```python
from build123d import *

# Parameters (mm, degrees)
EXTRUDE_1_DEPTH              = 14
SKETCH_2_R                   = 38
EXTRUDE_2_DEPTH              = 6
SKETCH_3_R                   = 31
EXTRUDE_3_DEPTH              = 28
SKETCH_4_R                   = 20
CUT_EXTRUDE_4_DEPTH          = 88.8179936
SKETCH_5_R                   = 2.5
CUT_EXTRUDE_5_DEPTH          = 79.689262292
HOLE_WIZARD_M8_1_D           = 9
HOLE_WIZARD_M8_1_CBORE_D     = 15
HOLE_WIZARD_M8_1_CBORE_DEPTH = 8
FILLET_1_R                   = 14


with BuildPart() as part:
    # 草圖1 → 伸長1 (new body)
    with BuildSketch(Plane(origin=(0, 0, 0), x_dir=(0, 0, -1), z_dir=(1, 0, 0))):
        with BuildLine():
            ThreePointArc((41.00892786, 41.00892786), (0, 52), (-41.00892786, 41.00892786))
            ThreePointArc((-41.00892786, 41.00892786), (-52, 0), (-41.00892786, -41.00892786))
            ThreePointArc((-41.00892786, -41.00892786), (0, -52), (41.00892786, -41.00892786))
            ThreePointArc((41.00892786, -41.00892786), (52, 0), (41.00892786, 41.00892786))
        make_face()
    extrude(amount=EXTRUDE_1_DEPTH)

    # 草圖2 → 伸長2 (add)
    with BuildSketch(Plane(origin=(14, 0, 0), x_dir=(0, 0, -1), z_dir=(1, 0, 0))):
        Circle(SKETCH_2_R)
    extrude(amount=EXTRUDE_2_DEPTH)

    # 草圖3 → 伸長3 (add)
    with BuildSketch(Plane.ZY):
        with Locations(Location((0, 0, 0), (0, 0, 180))):
            Circle(SKETCH_3_R)
    extrude(amount=EXTRUDE_3_DEPTH)

    # 草圖4 → 伸長4 (cut, through all)
    with BuildSketch(Plane(origin=(20, 0, 0), x_dir=(0, 0, -1), z_dir=(1, 0, 0))):
        Circle(SKETCH_4_R)
    extrude(amount=-CUT_EXTRUDE_4_DEPTH, mode=Mode.SUBTRACT)

    # 草圖5 → 伸長5 (cut, through all)
    with BuildSketch(Plane(origin=(0, 0, 0), x_dir=(1, 0, 0), z_dir=(0, 1, 0))):
        with Locations(Location((-18, 0, 0), (0, 0, 90))):
            Circle(SKETCH_5_R)
    extrude(amount=CUT_EXTRUDE_5_DEPTH, mode=Mode.SUBTRACT)

    # M8 六角承窩頭蓋螺釘的柱孔1 (through all)
    with Locations(Plane(origin=(20, 0, 0), x_dir=(0, 0, -1), z_dir=(1, 0, 0))):
        with Locations((29.69848481, 29.69848481), (29.69848481, -29.69848481), (-29.69848481, 29.69848481), (-29.69848481, -29.69848481)):
            CounterBoreHole(HOLE_WIZARD_M8_1_D / 2, HOLE_WIZARD_M8_1_CBORE_D / 2, HOLE_WIZARD_M8_1_CBORE_DEPTH)

    # 圓角1
    fillet_1_edges = [part.edges().sort_by_distance(p)[0] for p in [
        (7, 41.00892786, 41.00892786),
        (7, 41.00892786, -41.00892786),
        (7, -41.00892786, -41.00892786),
        (7, -41.00892786, 41.00892786),
    ]]
    fillet(fillet_1_edges, radius=FILLET_1_R)


solid = part.part
```
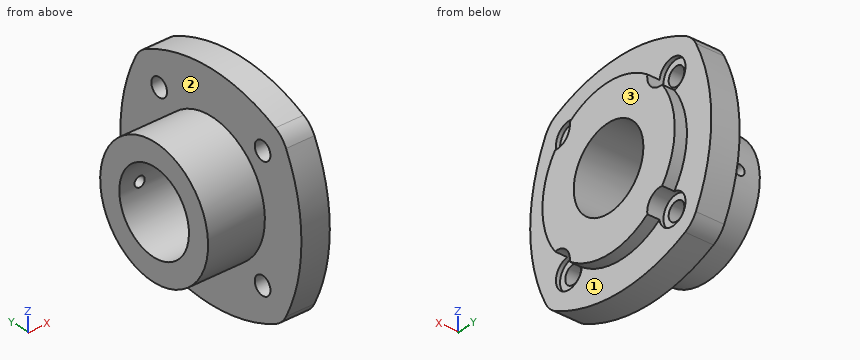
Could you check a few things on this model? Use its own coordinates, in mm. Face numbers are marked on the shaded views. A direction names the side the tool comes from. Give positions to 0.01 mm unless a question says otherwise; leave off trailing zeros. Loops run counter-clockwise (first coordinate to the right, second up) from the corner with the lowest first, then second, coordinate; pieces in that order, holes last. Notation, with made-up numbers: (50, -15.75) - (60, -15.75) arc R35 cw to (60, 16.25) - close; hole circle Ø2 at (-31.5, 80). An arc over 180 degrees is marked (long way). Answer in a Markdown table with one row per item. Add a question column.
Q1. Which directions (+Z, -Z, +X, -X, +Y, -Y) give clear straight access to the entire face, cutting with the end or side of a thin tool? Please do the marked faces 1, 2 and 3.
Q2. If we section it at A-A (y = 0): List the corners of the cut face in (x, z) for me.
Q3. Please list where these lines run through material, in increasing order: L1, parallel to Z at x = 7, y = -0.5; L2, parallel to Y at x = -3, z = 0; L3, parallel to X at y = 28, z = 0. Write a range as from..to.
Q4. If we section it at B-B (z = 0): List the corners of the cut face in (x, y) for me.
Q5. If we section it at C-C (y = -27.5): List the corners of the cut face in (x, z) for me, plus the area to 3 significant figures.
Q6. For pin 1 (12 mm diameter, centred on x = 1, y = 17, fed in from -Z); pin 2 (8 mm diameter, centred on x = -2.5, y = -39, fed in from -Z); pin 3 (11.5 mm diameter, centred on y = 29.7, z = 29.7, fed in from -X), each with a flat end and sliding along its axis, tell me the tip position at first contact or that it passes through.
Q7. If we section it at D-D (z = -17.5): List the corners of the cut face in (x, y) for me, plus the area to 3 significant figures.
The answers:
| question | item | result |
|---|---|---|
| 1 | face 1 | +X |
| 1 | face 2 | -X |
| 1 | face 3 | +Z, -Z, +X, +Y, -Y |
| 2 | outline | (-28, -31) - (0, -31) - (0, -52) - (14, -52) - (14, -38) - (20, -38) - (20, -20) - (-28, -20) - close; (-28, 20) - (20, 20) - (20, 38) - (14, 38) - (14, 52) - (0, 52) - (0, 31) - (-28, 31) - close |
| 3 | L1 | z = -52..-19.99, 19.99..52 |
| 3 | L2 | y = -31..-20, 20..31 |
| 3 | L3 | x = -28..-20.5, -15.5..20 |
| 4 | outline | (-28, -31) - (0, -31) - (0, -52) - (14, -52) - (14, -38) - (20, -38) - (20, -20) - (-28, -20) - close; (-28, 20) - (-20.5, 20) - (-20.5, 31) - (-28, 31) - close; (-15.5, 20) - (20, 20) - (20, 38) - (14, 38) - (14, 52) - (0, 52) - (0, 31) - (-15.5, 31) - close |
| 5 | outline | (-28, -14.31) - (0, -14.31) - (0, -25.77) - (12, -25.77) - (12, -22.53) - (20, -22.53) - (20, 22.53) - (12, 22.53) - (12, 25.77) - (0, 25.77) - (0, 14.31) - (-28, 14.31) - close; (0, -47.25) - (14, -47.25) - (14, -36.87) - (12, -36.87) - (12, -33.62) - (0, -33.62) - close; (0, 33.62) - (12, 33.62) - (12, 36.87) - (14, 36.87) - (14, 47.25) - (0, 47.25) - close |
| 5 | area | 2,150 mm^2 |
| 6 | pin 1 | stops at z = -51.26 |
| 6 | pin 2 | stops at z = -43.73 |
| 6 | pin 3 | stops at x = 0 |
| 7 | outline | (-28, -25.59) - (0, -25.59) - (0, -50.11) - (14, -50.11) - (14, -33.73) - (20, -33.73) - (20, -9.68) - (-28, -9.68) - close; (-28, 9.68) - (20, 9.68) - (20, 33.73) - (14, 33.73) - (14, 50.11) - (0, 50.11) - (0, 25.59) - (-28, 25.59) - close |
| 7 | area | 2,310 mm^2 |
